Read the model definition and answer for the solid it produces. Units are mm, in the model's axes. Face numbers are marked on the shaded views. A direction names the side the tool comes from. Coordinates: 2 decimals unless noted, no trailing zeros. Order: outer loops, then holes, each group sorted by start corner. A loop starts at its lowest first (then second) coordinate and runs counter-clockwise, first axis right, second up. Notation, with made-up numbers: (-22, -16.5) -> (-6, -16.5) arc R11 cw to (-6, -1.5) -> close; hole circle Ø1 at (-23.75, 58). An arc over 180 degrees is marked (long way). Use CSV: the item, a comma, the result in double quotes.
```python
from build123d import *

# Parameters (mm, degrees)
F2_SIZE  = 0.4
F3_SIZE  = 0.2
F4_R     = 0.6
F5_DEPTH = 8


with BuildPart() as f1:
    # F0 (on Right) → F1 (revolve)
    with BuildSketch(Plane.YZ):
        Polygon((0, 1.3), (0, 0), (18, 0), (18, 0.75), (10, 0.75), (10, 1), (8, 1), (8, 1.3), (6, 1.3), (6, 1), (3, 1), (3, 1.3), align=None)
    revolve(axis=Axis((0, 9, 0), (0, -1, 0)))

    # F2
    f2_edges = [f1.edges().sort_by_distance(p)[0] for p in [
        (0, 18, -0.75),
    ]]
    chamfer(f2_edges, length=F2_SIZE)

    # F3
    f3_edges = [f1.edges().sort_by_distance(p)[0] for p in [
        (0, 10, -1),
    ]]
    chamfer(f3_edges, length=F3_SIZE)

    # F4 (on face) → F5 (cut)
    with BuildSketch(Plane.XZ):
        Circle(F4_R)
    extrude(amount=-F5_DEPTH, mode=Mode.SUBTRACT)


solid = f1.part
```
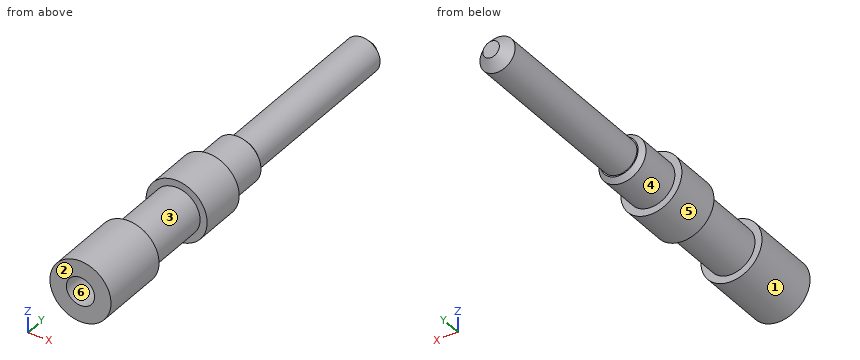
Item 1: Find section B-B, the plane y = 7.75. Give the vertices of the cut face in (x, z).
Return value:
outline,"circle Ø2.6 at (0, 0); hole circle Ø1.2 at (0, 0)"
Item 2: Find section C-C, the plane y = 15.25. Give the vertices of the cut face in (x, z).
Return value:
outline,"circle Ø1.5 at (0, 0)"
Item 3: Find section D-D, the plane y = 5. Give the vertices of the cut face in (x, z).
Return value:
outline,"circle Ø2 at (0, 0); hole circle Ø1.2 at (0, 0)"
Item 4: A tool of negligible diameter and unlimited length cuts with its end or side. For the marked faces 4, 5 and 6, from which of +Z, -Z, +X, -X, +Y, -Y can it reach the whole face along a straight path? Write none if from no direction.
Return value:
face 4,"+Y"
face 5,"+Y, -Y"
face 6,"-Y"
Item 5: Straight lines are drawn through the part: line 1 along Z through (x, y) = (0, 2.5); line 2 along Z through (x, y) = (0, 3.25); line 3 along Y through (x, z) = (1.25, -0.05). For each, find the intervals that lie inside material, in ascending order.
Return value:
line 1,"z = -1.3 to -0.6, 0.6 to 1.3"
line 2,"z = -1 to -0.6, 0.6 to 1"
line 3,"y = 0 to 3, 6 to 8"
Item 6: Find section A-A, the plane x = 0. Give the vertices of the cut face in (y, z).
Return value:
outline,"(0, -1.3) -> (3, -1.3) -> (3, -1) -> (6, -1) -> (6, -1.3) -> (8, -1.3) -> (8, -1) -> (9.8, -1) -> (10, -0.8) -> (10, -0.75) -> (17.6, -0.75) -> (18, -0.35) -> (18, 0.35) -> (17.6, 0.75) -> (10, 0.75) -> (10, 0.8) -> (9.8, 1) -> (8, 1) -> (8, 1.3) -> (6, 1.3) -> (6, 1) -> (3, 1) -> (3, 1.3) -> (0, 1.3) -> (0, 0.6) -> (8, 0.6) -> (8, -0.6) -> (0, -0.6) -> close"
Item 7: The mould has two halves that part along Y. Classify the marked faces 1, 2 and 3: +Y half, -Y half, draft (parallel to the pull), parting line (faces both ways), or undercut.
Return value:
face 1,"draft"
face 2,"-Y half"
face 3,"undercut"
Item 8: This flat-tipped pin is pushed along its axis until it touches: P1, Ø1, axis at x = -0.5, z = -1, coming from the +Y side. Where does it stop, or does it pass through?
Return value:
P1,"stops at y = 17.73"
